Read the model definition and answer for the solid it produces. Units are mm, in the model's axes. A direction names the side the tool comes from. Round coordinates to 2 decimals unless told otherwise and drop trailing zeros. Loops run counter-clockwise (first coordinate to the right, second up) from the corner with the lowest first, then second, coordinate; pieces in that order, holes last. Notation, with made-up numbers: M 41,14.5 L 49,14.5 A21 cw 49,28.5 Z; hole C 20.25,34 d9. An arc over 180 degrees is marked long. Write each question's results on one line, items separated by ' | '.
from build123d import *

# Parameters (mm, degrees)
F1_R      = 25
F1_R_2    = 24
F4_DEPTH  = 27.5
F5_R      = 25
F6_DEPTH  = 50
F7_R      = 22.5
F8_DEPTH  = 55
F9_R      = 21.5
F10_DEPTH = 20
F9_R_2    = 22.5
F11_DEPTH = 38.5
F13_DEPTH = 38.5


with BuildPart() as f2:
    # F2: sweep along a path in F0
    with BuildLine(Plane.YZ) as f2_path:
        Line((0, 0), (0, 200))
    # F1 (on Top) → F2 (sweep)
    with BuildSketch(Plane.XY):
        Circle(F1_R)
        Circle(F1_R_2, mode=Mode.SUBTRACT)
    sweep(path=f2_path.line)

    # F3 (on Right) → F4 (join, symmetric)
    with BuildSketch(Plane.YZ):
        Polygon((-27.5, 200), (-25, 200), (25, 200), (27.5, 200), (27.5, 203), (-27.5, 203), align=None)
    extrude(amount=F4_DEPTH, both=True)

    # F5 (on face) → F6 (join)
    with BuildSketch(Plane.XY.offset(203)):
        Circle(F5_R)
    extrude(amount=F6_DEPTH)

    # F7 (on face) → F8 (join)
    with BuildSketch(Plane.XY.offset(253)):
        Circle(F7_R)
    extrude(amount=F8_DEPTH)

    # F9 (on face) → F10 (cut)
    with BuildSketch(Plane(origin=(0, 27.5, 0), x_dir=(-1, 0, 0), z_dir=(0, 1, 0))):
        with Locations((0, 25)):
            Circle(F9_R)
    extrude(amount=-F10_DEPTH, mode=Mode.SUBTRACT)

    # F9 (on face) → F11 (join, symmetric)
    with BuildSketch(Plane(origin=(0, 27.5, 0), x_dir=(-1, 0, 0), z_dir=(0, 1, 0))):
        with Locations((0, 25)):
            Circle(F9_R_2)
        with Locations((0, 25)):
            Circle(F9_R, mode=Mode.SUBTRACT)
    extrude(amount=F11_DEPTH, both=True)

    # F12 (on face) → F13 (cut)
    with BuildSketch(Plane.XZ.offset(27.5)):
        with BuildLine():
            Line((-20, 175), (-20, 135))
            ThreePointArc((-20, 135), (0, 115), (20, 135))
            Line((20, 135), (20, 175))
            ThreePointArc((20, 175), (0, 195), (-20, 175))
        make_face()
    extrude(amount=-F13_DEPTH, mode=Mode.SUBTRACT)


solid = f2.part
Item 1: Straight lines are drawn through the part: line 1 (Z direction, x = 0, y = 17); line 2 (Z direction, x = 1.5, y = 10.5); line 3 (X direction, y = -2, z = 30). For each, find the intervals that lie inside material, in ascending order.
Outcome:
line 1: z = 2.5 to 3.5, 46.5 to 47.5, 200 to 308 | line 2: z = 2.55 to 3.55, 46.45 to 47.45, 200 to 308 | line 3: x = -24.92 to -23.92, -21.94 to -20.91, 20.91 to 21.94, 23.92 to 24.92
Item 2: The part is cut by section C-C (x = 12.5). State how many separate pieces and enclosed holes the cut face has, plus the area to 3 significant figures.
Outcome:
separate pieces: 3 | enclosed holes: 0 | area: 4,910 mm2
Item 3: The mould has two halves that part along X. Classify faces 1 (the face through (3.3, -11, 46.4)), 2 (the face through (-20.784, 44.957, 16.382)), 3 (the face through (-22, 66, 23)): pulls with the +X half, pulls with the -X half, needs draft (parallel to the pull), parting line crosses it, or undercut.
Outcome:
face 1: undercut | face 2: parting line crosses it | face 3: needs draft
Item 4: The part is cut by section B-B (z = 164). Determine the outline of the cut face in (x, y).
Outcome:
outline: M -20,-15 L -20,-13.27 A24 cw long 20,-13.27 L 20,-15 A25 ccw long Z
Item 5: The part is cut by section A-A (y = 0). Determine the outline of the cut face in (x, z), plus the area to 3 significant figures.
Outcome:
outline: M -27.5,200 L -25,200 L -25,0 L -24,0 L -24,200 L 24,200 L 24,0 L 25,0 L 25,200 L 27.5,200 L 27.5,203 L 25,203 L 25,253 L 22.5,253 L 22.5,308 L -22.5,308 L -22.5,253 L -25,253 L -25,203 L -27.5,203 Z; C 0,25 d45; hole C 0,25 d43 | area: 5,680 mm2
Item 6: Flat-ended cylindrical pins translate along their axes: pin 1 (2 mm diameter, centred on x = -8.5, z = 101.5, fed in from +Y); pin 2 (10 mm diameter, centred on y = 12, z = 79, fed in from +X); pin 3 (4 mm diameter, centred on x = -19, z = 211.5, fed in from -Y). Find the tip coordinate at first contact, or state that the pin passes through.
Outcome:
pin 1: stops at y = 23.85 | pin 2: stops at x = 24 | pin 3: stops at y = -18.33
Item 7: For faces 4 (the face through (0, 0, 308)), 5 (the face through (-8, -25, 200)), 6 (the face through (10.382, -19.961, 280.115)), 7 (the face through (0.1, -24.4, 195)), determine the directions among +Z, -Z, +X, -X, +Y, -Y from which every point of the face is accessible in a straight line to the end or side of a thin tool.
Outcome:
face 4: +Z, +X, -X, +Y, -Y | face 5: none | face 6: +Z | face 7: -Y
